Input: part model. Units: mm. Frame: model coordinates. Face numbers are marked on the shaded views. A direction names the side the tool comes from. Round coordinates to 2 decimals unless told otherwise and drop trailing zeros. Order: outer loops, then holes, each group sorted by start corner. A loop starts at its lowest first (then second) coordinate and runs counter-clockwise, first axis right, second up. Notation, with made-up numbers: (65, 88.25) -> (93, 88.25) arc R28 cw to (93, 127.25) -> close; hole circle Ø6 at (60.5, 20.5). An arc over 180 degrees is marked (long way). Use a Markdown table: item, result.
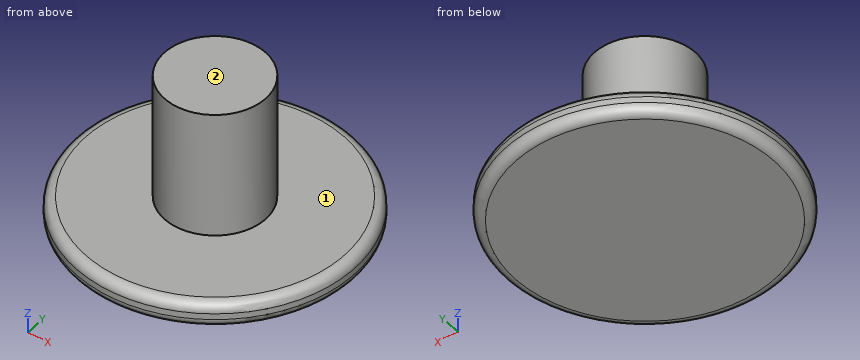
from build123d import *

# Parameters (mm, degrees)
F0_R     = 11
F1_DEPTH = 2
F2_R     = 4.0005
F3_DEPTH = 12
F4_R     = 0.762


with BuildPart() as f1:
    # F0 (on Top) → F1 (new body)
    with BuildSketch(Plane.XY):
        Circle(F0_R)
    extrude(amount=F1_DEPTH)

    # F2 (on Top) → F3 (join)
    with BuildSketch(Plane.XY):
        Circle(F2_R)
    extrude(amount=F3_DEPTH)

    # F4
    f4_edges = [f1.edges().sort_by_distance(p)[0] for p in [
        (-11, 0, 2),
        (11, 0, 1),
        (-11, 0, 0),
    ]]
    fillet(f4_edges, radius=F4_R)


solid = f1.part
1) Set-up query: the marked faces 1 and 2. Return all of +Z, -Z, +X, -X, +Y, -Y with unobstructed straight access to the full face (end or side cutting, diameter ignored); none if empty.
Results found:
| item | result |
|---|---|
| face 1 | +Z |
| face 2 | +Z, +X, -X, +Y, -Y |
2) Pin query (flat end, axial travel): pin 1 Ø3 at (y, z) = (0, 9) entering from -X; pin 2 Ø8 at (x, y) = (8.5, 1.5) entering from +Z; pin 3 Ø12 at (x, y) = (6, -1) entering from +Z; pin 4 Ø6 at (x, z) = (7, 3.5) entering from -Y. Return the tip coordinate at first contact, or that it passes through.
Results found:
| item | result |
|---|---|
| pin 1 | stops at x = -4 |
| pin 2 | stops at z = 2 |
| pin 3 | stops at z = 12 |
| pin 4 | stops at y = -9.86 |
3) Cut plane A-A on x = 0. Return loops of the section in (y, z).
Results found:
| item | result |
|---|---|
| outline | (-11, 0.76) arc R0.76 ccw to (-10.24, 0) -> (10.24, 0) arc R0.76 ccw to (11, 0.76) -> (11, 1.24) arc R0.76 ccw to (10.24, 2) -> (4, 2) -> (4, 12) -> (-4, 12) -> (-4, 2) -> (-10.24, 2) arc R0.76 ccw to (-11, 1.24) -> close |
4) Line query: L1, parallel to Z at x = -2, y = -5; L2, parallel to Y at x = 0, z = 3.5; L3, parallel to X at y = 2.25, z = 2.5. Output: solid intervals per line, ascending. Write a range as [from, to].
Results found:
| item | result |
|---|---|
| L1 | z = [0, 2] |
| L2 | y = [-4, 4] |
| L3 | x = [-3.31, 3.31] |
5) Cut plane C-C on z = 6.5. Return loops of the section in (x, y), and give its area (3 significant figures).
Results found:
| item | result |
|---|---|
| outline | circle Ø8 at (0, 0) |
| area | 50.3 mm² |
